Source: three-view drawing plus pictorial views. Frame: mm from the lowest corner of the part. A direction names the side the tool comes from. Coordinates: 2 decimals unless noted, no trailing zeros. Loops run counter-clockwise (first coordinate to the right, second up) from the corner with the lowest first, then second, coordinate; pieces in that order, holes last. Notation, with made-up numbers: (28.5, 8.5) - (33.5, 8.5) arc R22 ccw to (33.5, 40.5) - close; hole circle Ø1 at (-7.75, 25). An arc over 180 degrees is marked (long way). Return JSON: item names as keys, results as strings.
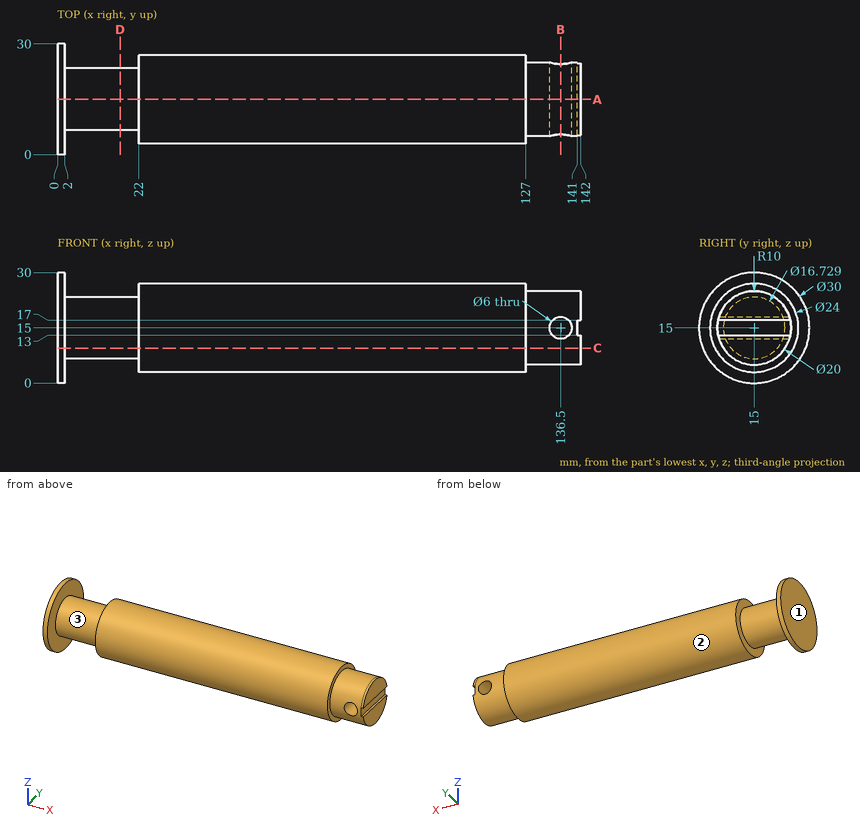
Item 1: Ray query, probe 1 along X at (y, z) = (17.75, 5.75); probe 2 along Z at (x, y) = (136.5, 15); probe 3 along X at (y, z) = (20.5, 15). Return the intervals inside material, ascending. Write a range as from..to.
Worked out:
{"probe 1": "0..2, 22..142", "probe 2": "5..12, 18..25", "probe 3": "0..133.5, 139.5..141"}
Item 2: Section query A-A, the plane y = 15. Return loops of the section in (x, z) (1 decimal).
Worked out:
{"outline": "(0, 0) - (2, 0) - (2, 6.6) - (22, 6.6) - (22, 3) - (127, 3) - (127, 5) - (142, 5) - (142, 13) - (141, 13) - (141, 17) - (142, 17) - (142, 25) - (127, 25) - (127, 27) - (22, 27) - (22, 23.4) - (2, 23.4) - (2, 30) - (0, 30) - close; hole circle Ø6 at (136.5, 15)"}
Item 3: Section query B-B, the plane x = 136.5. Return loops of the section in (y, z), and give its area (3 significant figures).
Worked out:
{"outline": "(5.46, 12) arc R10 ccw to (24.54, 12) - close; (5.46, 18) - (24.54, 18) arc R10 ccw to start", "area": "196 mm^2"}
Item 4: Section query D-D, the plane x = 17. Return loops of the section in (y, z) (1 decimal).
Worked out:
{"outline": "circle Ø16.7 at (15, 15)"}
Item 5: Reachability of the marked faces 1, 2 and 3 from +Z, -Z, +X, -X, +Y, -Y: full face, straight path, thin tool, end or side. Return the list, or none.
Worked out:
{"face 1": "+Z, -Z, -X, +Y, -Y", "face 2": "+X", "face 3": "none"}
Item 6: First-contact query: pin 1 Ø1.5 at (x, y) = (16, 15.5) entering from -Z; pin 2 Ø1.1 at (x, y) = (141.5, 14.5) entering from +Z; pin 3 Ø4 at (x, y) = (79.5, 7.5) entering from -Z (1 decimal); pin 4 Ø10 at (y, z) = (14.5, 15) entering from -X. Flat tips, straight axial feed; report the tip coordinate or a pass-through.
Worked out:
{"pin 1": "z = 6.64", "pin 2": "z = 25", "pin 3": "z = 4.3", "pin 4": "x = 0"}
Item 7: Section query C-C, the plane z = 9.5. Return loops of the section in (x, y) (1 decimal).
Worked out:
{"outline": "(0, 1) - (2, 1) - (2, 8.7) - (22, 8.7) - (22, 4.3) - (127, 4.3) - (127, 6.6) - (142, 6.6) - (142, 23.4) - (127, 23.4) - (127, 25.7) - (22, 25.7) - (22, 21.3) - (2, 21.3) - (2, 29) - (0, 29) - close"}
